For this review, take the finished solid that the model builds, in its own axes (mm). Give positions to 0.01 mm unless a question says otherwise; leave off trailing zeros. Order: outer loops, then holes, each group sorted by start corner. A loop starts at its lowest first (then second) coordinate and runs counter-clockwise, first axis right, second up. Notation, with made-up numbers: (45, -34) -> (94, -34) arc R21 cw to (94, -18) -> close; hole circle Ø11 at (48.5, -9). An arc over 180 degrees is marked (long way). Return JSON: item names as keys, results as strings. Group by question number.
1) Insertion check: P1, Ø4.5, axis at x = 40, y = 20, coming from the -Z side; P2, Ø2, axis at x = 43, z = 21.5, coming from the -Y side; P3, Ø1, axis at x = 38, z = 19.5, coming from the +Y side; P4, Ø1.2, axis at x = 41, y = 20, coming from the -Z side. Each pin has a flat end and moves straight along its axis. Give the tip position at first contact, or say it passes through.
2) The part is to be moulded in two halves that separate along X. For faces 1 (the face through (40, 20, 49.3)), 2 (the face through (40, 20, 35)), 3 (the face through (40, 18, 17)), 4 (the face through (37.05, 17.3, 23.32)), say which applies: released by +X, released by -X, zero draft, split by the parting line, or undercut.
3) Add section A-A (z = 6.5). Give the boundary of the cut face in (x, y).
4) Add section B-B (z = 42.5). Give the boundary of the cut face in (x, y).
5) To check wall thickness, follow line 1 along Y through (x, z) = (40, 15.5); line 2 along X through (y, z) = (19, 10.5); line 3 along Y through (x, z) = (41.25, 31.5). State the ranges of each line that lie inside material, in increasing order.
Autodesk Fusion 360 part; units mm, degrees
sketch "Sketch1" plane through (0, 0, 0) normal (0, 0, 1) x (1, 0, 0)
  circle A0 centre (40, 20) radius 2
  circle A1 centre (40, 20) radius 4
  dimension "d1" = 4
  dimension "d2" = 8
extrude "Extrude1" add sketch "Sketch1" along normal blind 35 makes body 1
sketch "Sketch2" plane through (0, 0, 35) normal (0, 0, 1) x (-1, 0, 0)
  circle A0 centre (-40, -20) radius 2
  circle A1 centre (-40, -20) radius 4
  circle A2 centre (-40, -20) radius 4
  circle A3 centre (-40, -20) radius 2
  dimension "d5" = 8
extrude "Extrude2" add sketch "Sketch2" along normal blind 14.3 separate body contours A0 A3 makes body 2
extrude "Extrude3" add 1 faces at (43.311, 19.7019, 35) along direction (0, 0, 1) blind 14.3 on bodies 1 bodies 1 2
fillet "Fillet1" radius 2 1 edges at (36.2707, 18.5535, 49.3) on bodies 1
Evaluation:
{
 "1": {"P1": "z = 0", "P2": "y = 16.54", "P3": "y = 23.71", "P4": "z = 35"},
 "2": {"face 1": "zero draft", "face 2": "undercut", "face 3": "undercut", "face 4": "split by the parting line"},
 "3": {"outline": "circle Ø8 at (40, 20); hole circle Ø4 at (40, 20)"},
 "4": {"outline": "circle Ø8 at (40, 20)"},
 "5": {"line 1": "16 to 18, 22 to 24", "line 2": "36.13 to 38.27, 41.73 to 43.87", "line 3": "16.2 to 18.44, 21.56 to 23.8"}
}
